Source: CAD feature listing. Evaluate the final solid. Frame: model axes, mm. Face numbers are marked on the shaded views. A direction names the side the tool comes from. Round coordinates to 2 decimals unless told otherwise and drop trailing zeros. Write each loop counter-clockwise with the first axis right and the second up, starting at its lowest first coordinate (ties: lowest second). Pieces come first, ordered by that corner, then holes. Notation, with made-up numbers: (40.5, 87) -> (63.5, 87) arc R22 ccw to (63.5, 112) -> close; hole circle Ø2 at (-25, 59). An arc over 180 degrees is marked (long way). Put each result on its own line as item: value.
```python
from build123d import *

# Parameters (mm, degrees)
F0_W      = 32
F0_H      = 13
F1_DEPTH  = 113
F2_W      = 35
F2_H      = 32
F3_DEPTH  = 17
F4_W      = 25
F4_H      = 30.1287648325
F4_H_2    = 18.8096150512
F4_W_2    = 26
F4_H_3    = 47.1287648325
F5_DEPTH  = 32.001
F6_R      = 5.5
F7_DEPTH  = 13.001
F8_R      = 5.5
F9_DEPTH  = 13.001
F10_R     = 6.5
F11_DEPTH = 87.001


with BuildPart() as f1:
    # F0 (on Right) → F1 (new body)
    with BuildSketch(Plane.YZ):
        with Locations((16, 6.5)):
            Rectangle(F0_W, F0_H)
        with BuildLine():
            Line((0, 60.1287648325), (0, 13))
            Line((0, 13), (32, 13))
            Line((32, 13), (32, 60.1287648325))
            ThreePointArc((32, 60.1287648325), (16, 64), (0, 60.1287648325))
        make_face()
    extrude(amount=F1_DEPTH)

    # F2 (on face) → F3 (cut)
    with BuildSketch(Plane(origin=(0, 0, 0), x_dir=(1, 0, 0), z_dir=(0, 0, -1))):
        with Locations((56.5, -16)):
            Rectangle(F2_W, F2_H)
    extrude(amount=-F3_DEPTH, mode=Mode.SUBTRACT)

    # F4 (on face) → F5 (cut, through all)
    with BuildSketch(Plane.XZ):
        with Locations((56.5, 45.0643824163)):
            Rectangle(F4_W, F4_H)
        with Locations((56.5, 69.5335723582)):
            Rectangle(F4_W, F4_H_2)
        with Locations((100, 36.5643824163)):
            Rectangle(F4_W_2, F4_H_3)
        with Locations((100, 69.5335723582)):
            Rectangle(F4_W_2, F4_H_2)
        with Locations((13, 69.5335723582)):
            Rectangle(F4_W_2, F4_H_2)
        with Locations((13, 36.5643824163)):
            Rectangle(F4_W_2, F4_H_3)
    extrude(amount=-F5_DEPTH, mode=Mode.SUBTRACT)

    # F6 (on face) → F7 (cut, through all)
    with BuildSketch(Plane.XY.offset(13)):
        Polygon((113, 0), (113, 16), (100, 0), align=None)
        with Locations((100, 19)):
            Circle(F6_R)
    extrude(amount=-F7_DEPTH, mode=Mode.SUBTRACT)

    # F8 (on face) → F9 (cut, through all)
    with BuildSketch(Plane.XY.offset(13)):
        with Locations((13, 19)):
            Circle(F8_R)
        Polygon((0, 16), (0, 0), (13, 0), align=None)
    extrude(amount=-F9_DEPTH, mode=Mode.SUBTRACT)

    # F10 (on face) → F11 (cut, through all)
    with BuildSketch(Plane.YZ.offset(87)):
        with Locations((16, 46)):
            Circle(F10_R)
    extrude(amount=-F11_DEPTH, mode=Mode.SUBTRACT)


solid = f1.part
```
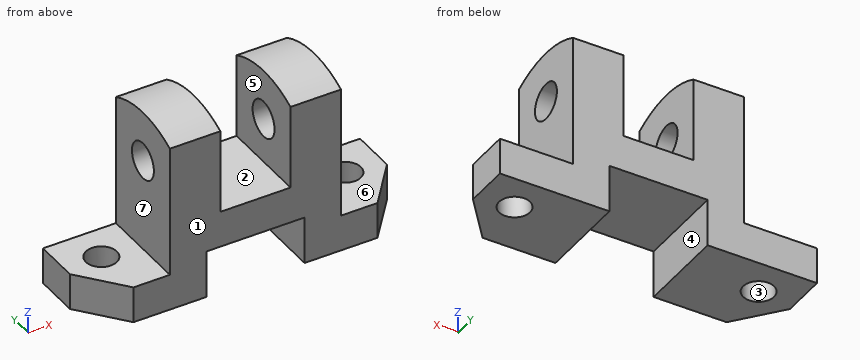
Q1. Cut plane D-D on z = 46. Output: boundary loops of the cut face in (x, y), and give its area (3 significant figures).
Ans:
outline: (26, 0) -> (44, 0) -> (44, 9.5) -> (26, 9.5) -> close; (26, 22.5) -> (44, 22.5) -> (44, 32) -> (26, 32) -> close; (69, 0) -> (87, 0) -> (87, 9.5) -> (69, 9.5) -> close; (69, 22.5) -> (87, 22.5) -> (87, 32) -> (69, 32) -> close
area: 684 mm^2
Q2. Pin query (flat end, axial travel): pin 1 (8 mm diameter, centred on y = 16, z = 46, fed in from +X); pin 2 (16 mm diameter, centred on y = 21.5, z = 51, fed in from -X); pin 3 (4 mm diameter, centred on x = 36.5, y = 19.5, fed in from +Z); pin 4 (8.5 mm diameter, centred on y = 9.5, z = 7, fed in from -X). Return the tip coordinate at first contact, or that it passes through.
Ans:
pin 1: passes through
pin 2: stops at x = 26
pin 3: stops at z = 63.97
pin 4: stops at x = 1.83
Q3. Cut plane C-C on x = 81. Output: boundary loops of the cut face in (y, z).
Ans:
outline: (0, 0) -> (32, 0) -> (32, 60.13) arc R35 ccw to (0, 60.13) -> close; hole circle Ø13 at (16, 46)
Q4. Cut plane B-B on z = 15.5. Output: boundary loops of the cut face in (x, y).
Ans:
outline: (26, 0) -> (39, 0) -> (39, 32) -> (26, 32) -> close; (74, 0) -> (87, 0) -> (87, 32) -> (74, 32) -> close
Q5. Cut plane A-A on z = 7.5. Output: boundary loops of the cut face in (x, y).
Ans:
outline: (0, 16) -> (13, 0) -> (39, 0) -> (39, 32) -> (0, 32) -> close; (74, 0) -> (100, 0) -> (113, 16) -> (113, 32) -> (74, 32) -> close; hole circle Ø11 at (13, 19); hole circle Ø11 at (100, 19)
Q6. Reachability of the marked faces 4, 5, 6 and 7 from +Z, -Z, +X, -X, +Y, -Y: full face, straight path, thin tool, end or side. Return the list, or none.
Ans:
face 4: -Z, +Y, -Y
face 5: +Z, +Y, -Y
face 6: +Z, +X, +Y, -Y
face 7: +Z, -X, +Y, -Y
Q7. Material intervals for line 1 (Y direction, x = 100, z = 7); line 2 (X direction, y = 20, z = 35); line 3 (Z direction, x = 81, y = 16), sorted ascending. Write a range as [from, to].
Ans:
line 1: y = [0, 13.5], [24.5, 32]
line 2: x = [26, 44], [69, 87]
line 3: z = [0, 39.5], [52.5, 64]
Q8. Draft query along Y for the marked faces 1, 2 and 3. Return one class per face: +Y half, -Y half, draft (parallel to the pull), parting line (faces both ways), or undercut.
Ans:
face 1: -Y half
face 2: draft
face 3: undercut
